Could you check a few things on this model? Use its own coordinates, in mm. A direction names the side the tool comes from. Give positions to 0.01 mm unless a question says otherwise; leave off trailing zeros. Loops run counter-clockwise (first coordinate to the right, second up) from the corner with the lowest first, then second, coordinate; pieces in that order, holes last. Notation, with made-up numbers: (-30.5, 85.25) -> (27.5, 85.25) arc R16 cw to (27.5, 105.25) -> close; hole circle Ø10 at (-38.5, 52.25). An arc over 180 degrees is marked (long way). Write each question's results on one line, items separated by ' | '. Start each with the question number.
Q1. If I drill on line 1 along X through (y, z) = (-65.5, 3); line 2 along Y through (x, z) = (-92, 8); line 3 along Y through (x, z) = (-53.5, 5.5), over which ranges is the centre line in solid material (lowest first)?
Q2. Will this pin go through, and if not, where does the flat tip stop? P1, Ø6, axis at x = -131.5, z = 2.5, coming from the -Y side.
Q3. If we section it at B-B, the plane x = -60: List the corners of the cut face in (y, z) for me, plus the area to 3 significant figures.
Q4. If we section it at A-A, the plane x = -75: List the corners of the cut face in (y, z) for me.
Q5. If we section it at D-D, the plane x = -44: List the corners of the cut face in (y, z) for me, plus the area to 3 significant figures.
Q6. If we section it at C-C, the plane y = -96.5: List the corners of the cut face in (x, z) for me, plus the area to 3 significant figures.
Q7. We'd pull the mould along Y, two halves only. Please class faces 1 (the face through (-150, -20, 5)), 2 (the face through (-48.797, -48.007, 4.786)), 3 (the face through (-74, 0, 5)): released by +Y, released by -Y, zero draft, split by the parting line, or undercut.
Q8. Which directions (+Z, -Z, +X, -X, +Y, -Y) give clear straight access to the entire face, cutting with the end or side of a thin tool? Please do faces 4 (the face through (0, -20, 5)), 5 (the face through (-45.92, -65.14, 5.07)), 6 (the face through (-75, -45, 5)).
from build123d import *
from OCP.BRepFilletAPI import BRepFilletAPI_MakeChamfer

# Parameters (mm, degrees)
SKETCH1_W           = 57.5
SKETCH1_H           = 30
BOSS_EXTRUDE1_DEPTH = 10
CHAMFER1_SIZE       = 10
CHAMFER1_SIZE_2     = 0.648423639
FILLET1_R           = 10


# Some blends are built 0.0001 mm under size
with BuildPart() as part:
    # Sketch1 → Boss-Extrude1 (new body)
    with BuildSketch(Plane.XY):
        with BuildLine():
            Line((0, -40), (0, 0))
            Line((0, 0), (-150, 0))
            Line((-150, 0), (-150, -40))
            ThreePointArc((-150, -40), (-75, -115), (0, -40))
        make_face()
        with Locations((-75, -60)):
            Rectangle(SKETCH1_W, SKETCH1_H, mode=Mode.SUBTRACT)
    extrude(amount=BOSS_EXTRUDE1_DEPTH)

    # Chamfer1
    chamfer1_edges_1 = [part.edges().sort_by_distance(p)[0] for p in [
        (-46.25, -60, 10),
    ]]
    chamfer1_side_1 = [part.faces().sort_by_distance(p)[0] for p in [
        (-46.25, -60, 9.987031527),
    ]]
    chamfer1_edges_2 = [part.edges().sort_by_distance(p)[0] for p in [
        (-103.75, -60, 10),
    ]]
    chamfer1_side_2 = [part.faces().sort_by_distance(p)[0] for p in [
        (-103.75, -60, 9.987031527),
    ]]
    chamfer1 = BRepFilletAPI_MakeChamfer(part.part.solid().wrapped)
    for e in chamfer1_edges_1:
        chamfer1.Add(CHAMFER1_SIZE - 0.0001, CHAMFER1_SIZE_2 - 0.0001, e.wrapped, chamfer1_side_1[0].wrapped)
    for e in chamfer1_edges_2:
        chamfer1.Add(CHAMFER1_SIZE - 0.0001, CHAMFER1_SIZE_2 - 0.0001, e.wrapped, chamfer1_side_2[0].wrapped)
    add(Compound.cast(chamfer1.Shape()), mode=Mode.REPLACE)  # a hair under: the kernel refuses the full size

    # Fillet1
    # the kernel refuses this fillet: 10 mm, written as the material it adds along each edge
    with BuildSketch(Plane(origin=(-47.867429584, -45, -24.947523565), x_dir=(-0.9979049426006561, 0, 0.06469718334812755), z_dir=(0.06469718334812756, 0, 0.9979049426006562))) as fillet1_piece_1_section:
        with BuildLine():
            CenterArc((FILLET1_R, FILLET1_R), FILLET1_R, 180, 90)
            Line((0, FILLET1_R), (0, 0))
            Line((0, 0), (FILLET1_R, 0))
        make_face()
    fillet1_piece_1 = extrude(amount=60.020894349, mode=Mode.PRIVATE)
    fillet1_piece_1 = split(fillet1_piece_1, bisect_by=Plane(origin=(-48.707082499, -46.782935943, 10), z_dir=(0, 0, -1)), keep=Keep.TOP, mode=Mode.PRIVATE)
    fillet1_piece_1 = split(fillet1_piece_1, bisect_by=Plane(origin=(-48.707082499, -46.782935943, 0), z_dir=(0, 0, 1)), keep=Keep.TOP, mode=Mode.PRIVATE)
    add(fillet1_piece_1)
    with BuildSketch(Plane(origin=(-102.132570416, -45, -24.947523565), x_dir=(0.9979049426006561, 0, 0.06469718334812756), z_dir=(-0.06469718334812756, 0, 0.9979049426006562))) as fillet1_piece_2_section:
        with BuildLine():
            CenterArc((FILLET1_R, -FILLET1_R), FILLET1_R, 90, 90)
            Line((0, -FILLET1_R), (0, 0))
            Line((0, 0), (FILLET1_R, 0))
        make_face()
    fillet1_piece_2 = extrude(amount=60.020894349, mode=Mode.PRIVATE)
    fillet1_piece_2 = split(fillet1_piece_2, bisect_by=Plane(origin=(-101.292917501, -46.782935943, 10), z_dir=(0, 0, -1)), keep=Keep.TOP, mode=Mode.PRIVATE)
    fillet1_piece_2 = split(fillet1_piece_2, bisect_by=Plane(origin=(-101.292917501, -46.782935943, 0), z_dir=(0, 0, 1)), keep=Keep.TOP, mode=Mode.PRIVATE)
    add(fillet1_piece_2)


solid = part.part
Final values:
1) line 1: x = -145.53 to -103.94, -46.06 to -4.47 | line 2: y = -113.05 to -75, -45 to 0 | line 3: y = -111.85 to -75, -45.29 to 0
2) P1: stops at y = -92.56
3) outline: (-113.48, 0) -> (-75, 0) -> (-75, 10) -> (-113.48, 10) -> close; (-45, 0) -> (0, 0) -> (0, 10) -> (-45, 10) -> close | area: 835 mm²
4) outline: (-115, 0) -> (-75, 0) -> (-75, 10) -> (-115, 10) -> close; (-45, 0) -> (0, 0) -> (0, 10) -> (-45, 10) -> close
5) outline: (-108.29, 0) -> (0, 0) -> (0, 10) -> (-108.29, 10) -> close | area: 1,080 mm²
6) outline: (-124.32, 0) -> (-25.68, 0) -> (-25.68, 10) -> (-124.32, 10) -> close | area: 986 mm²
7) face 1: zero draft | face 2: undercut | face 3: released by +Y
8) face 4: +Z, -Z, +X, +Y, -Y | face 5: +Z | face 6: +Z, -Z
